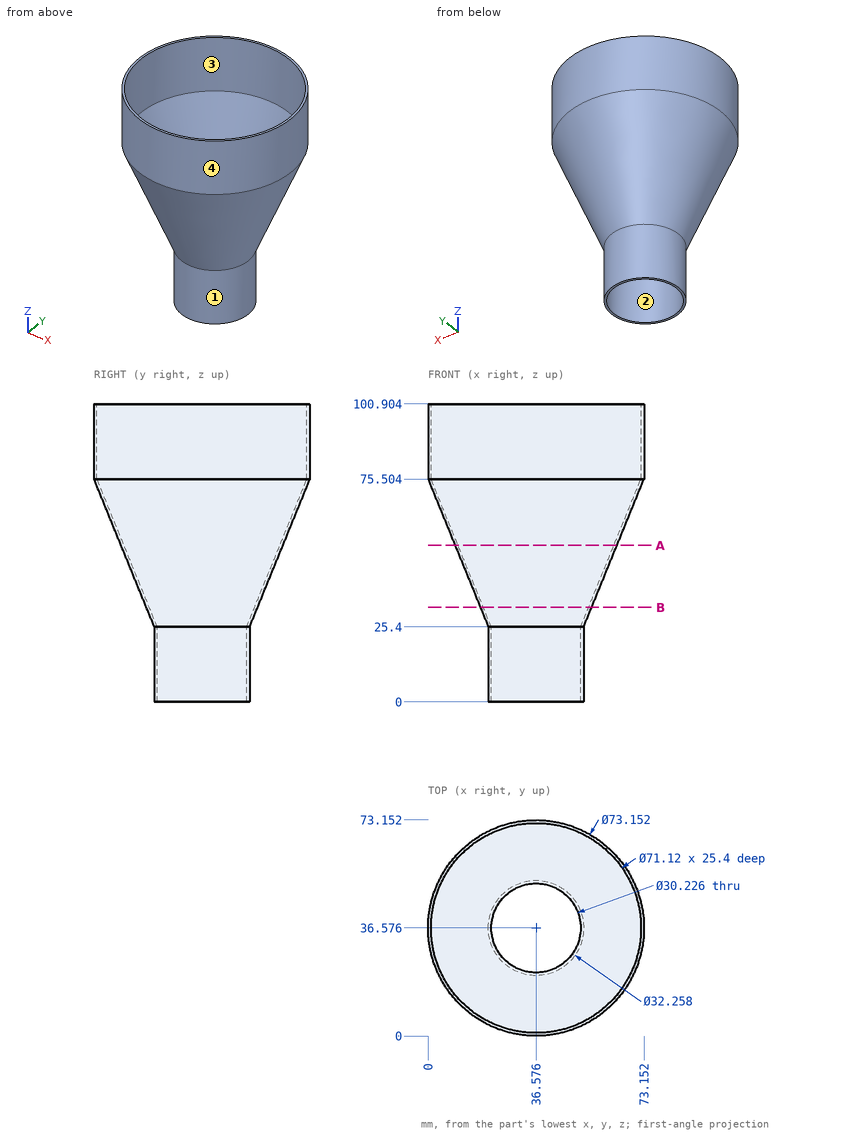
Print and shaded views of the part. All mm, measured from the part's lowest x, y and z. A direction names the side the tool comes from. Round coordinates to 2 decimals unless told otherwise and drop trailing zeros. Write each loop counter-clockwise with the first axis right and the second up, starting at its lowest first coordinate (ties: lowest second). Pieces come first, ordered by that corner, then holes. Notation, with made-up numbers: (58.25, -3.75) -> (110.25, -3.75) arc R17 ccw to (110.25, 13.25) -> close; hole circle Ø11 at (2.5, -36). An arc over 180 degrees is marked (long way). Return JSON: item names as keys, results as strings. Group by question number.
Q1. Saw through at B-B on z = 32. Write the cut outline in (x, y) (1 decimal), plus the area to 3 significant figures.
Q2. Which spindle directions (+Z, -Z, +X, -X, +Y, -Y) get a long thin tool onto all of the face, cutting with end or side? Do the marked faces 1 and 2. Say none if no direction does.
Q3. Saw through at A-A on z = 53. Write the cut outline in (x, y).
Q4. Mould opens along Y. For the marked faces 3 and 4 say: pulls with the +Y half, pulls with the -Y half, needs draft (parallel to the pull), parting line crosses it, or undercut.
Q5. Probe L1, parallel to X at y = 27, z = 40 (1 decimal); L2, parallel to Y at x = 60, z = 63.5; L3, parallel to X at y = 28.5, z = 89 (1 decimal). List the from-to ranges inside material, lowest first. Write a range as [from, to].
Q6. Pin check, flat tips, straight feed: pin 1 (5 mm diameter, centred on y = 30.5, z = 41.5, fed in from +X); pin 2 (3 mm diameter, centred on x = 12.5, y = 59, fed in from +Z) (1 decimal); pin 3 (1.5 mm diameter, centred on y = 10.5, z = 65, fed in from -X) (1 decimal); pin 4 (18 mm diameter, centred on x = 36.58, y = 36.58, fed in from +Z). Stop position of each tip, or through.
Answer:
{
 "1": {"outline": "circle Ø37.6 at (36.6, 36.6); hole circle Ø35.6 at (36.6, 36.6)", "area": "117 mm2"},
 "2": {"face 1": "-Z", "face 2": "+Z, -Z"},
 "3": {"outline": "circle Ø54.78 at (36.58, 36.58); hole circle Ø52.75 at (36.58, 36.58)"},
 "4": {"face 3": "undercut", "face 4": "parting line crosses it"},
 "5": {"L1": "[16.7, 17.8], [55.3, 56.5]", "L2": "[15.25, 16.79], [56.36, 57.9]", "L3": "[0.9, 1.9], [71.2, 72.2]"},
 "6": {"pin 1": "x = 59.66", "pin 2": "z = 72.7", "pin 3": "x = 16.4", "pin 4": "through"}
}
